```python
from build123d import *

# Parameters (mm, degrees)
SKETCH1_R           = 48.26
SKETCH1_R_2         = 1.1303
SKETCH1_R_3         = 17.4625
SKETCH1_R_4         = 3.175
BOSS_EXTRUDE1_DEPTH = 3.175


with BuildPart() as part:
    # Sketch1 → Boss-Extrude1 (new body)
    with BuildSketch(Plane(origin=(0, 0, 0), x_dir=(0, 0, -1), z_dir=(1, 0, 0))):
        Circle(SKETCH1_R)
        with Locations((0, 45.085)):
            Circle(SKETCH1_R_2, mode=Mode.SUBTRACT)
        with Locations((31.87990923, 31.87990923)):
            Circle(SKETCH1_R_2, mode=Mode.SUBTRACT)
        with Locations((45.085, 0)):
            Circle(SKETCH1_R_2, mode=Mode.SUBTRACT)
        with Locations((31.87990923, -31.87990923)):
            Circle(SKETCH1_R_2, mode=Mode.SUBTRACT)
        with Locations((0, -45.085)):
            Circle(SKETCH1_R_2, mode=Mode.SUBTRACT)
        with Locations((-31.87990923, -31.87990923)):
            Circle(SKETCH1_R_2, mode=Mode.SUBTRACT)
        with Locations((-45.085, 0)):
            Circle(SKETCH1_R_2, mode=Mode.SUBTRACT)
        with Locations((-31.87990923, 31.87990923)):
            Circle(SKETCH1_R_2, mode=Mode.SUBTRACT)
        Circle(SKETCH1_R_3, mode=Mode.SUBTRACT)
        with Locations((9.720159182, 23.466540126)):
            Circle(SKETCH1_R_4, mode=Mode.SUBTRACT)
        with Locations((23.466540126, -9.720159182)):
            Circle(SKETCH1_R_4, mode=Mode.SUBTRACT)
        with Locations((-9.720159182, -23.466540126)):
            Circle(SKETCH1_R_4, mode=Mode.SUBTRACT)
        with Locations((-23.466540126, 9.720159182)):
            Circle(SKETCH1_R_4, mode=Mode.SUBTRACT)
    extrude(amount=BOSS_EXTRUDE1_DEPTH)


solid = part.part
```
Check sheet for the modelled part. Datum: model origin and axes. Units: mm. Round coordinates to 2 decimals unless told otherwise and drop trailing zeros. Loops run counter-clockwise (first coordinate to the right, second up) from the corner with the lowest first, then second, coordinate; pieces in that order, holes last. Notation, with made-up numbers: (-17, -1.5) -> (2, -1.5) arc R18 cw to (2, 28.5) -> close; hole circle Ø8 at (38, 27.25). An arc over 180 degrees is marked (long way). Write item = value, one per line. Start each with the question number.
1) Sectioned sample at D-D, the plane z = -23.5. Record the cut outline in (x, y) (3 decimals).
2) Release check for a two-part mould opening along Y. For faces 1 (the flat face through (0, -21, 1)), 2 (the cylindrical face through (1.57, 14.5, -46.03)), 3 (the cylindrical face through (1.57, -30.93, 31.27)), 4 (the cylindrical face through (1.565, -43.964, 0.147)) record: released by +Y, released by -Y, zero draft, split by the parting line, or undercut.
3) Gauge pin test, flat ends, axial feed: pin 1 Ø2 at (y, z) = (-31.88, -31.88) entering from +X; pin 2 Ø1.5 at (x, y) = (2.5, 21.5) entering from -Z; pin 3 Ø1 at (x, y) = (2, 15.5) entering from -Z. Record the tip position at first contact, or that the pin passes through.
4) Sectioned sample at A-A, the plane z = 0. Record the cut outline in (x, y) (1 decimal).
5) Sectioned sample at C-C, the plane x = 2.2. State how many separate pieces and enclosed holes the cut face has, plus the area to 3 significant figures.
6) Thickness scan on probe 1 along Y at (x, z) = (1.9, 0); probe 2 along Y at (x, z) = (2.3, 31); probe 3 along Z at (x, y) = (2.15, -7.5). Record the ranges inside material, lowest first.
Results are:
q1.outline = (0, -42.152) -> (3.175, -42.152) -> (3.175, -12.895) -> (0, -12.895) -> close; (0, -6.545) -> (3.175, -6.545) -> (3.175, 42.152) -> (0, 42.152) -> close
q2.face_1 = zero draft
q2.face_2 = split by the parting line
q2.face_3 = undercut
q2.face_4 = undercut
q3.pin_1 = through
q3.pin_2 = -43.57
q3.pin_3 = -45.87
q4.outline = (0, -48.3) -> (3.2, -48.3) -> (3.2, -46.2) -> (0, -46.2) -> close; (0, -44) -> (3.2, -44) -> (3.2, -17.5) -> (0, -17.5) -> close; (0, 17.5) -> (3.2, 17.5) -> (3.2, 44) -> (0, 44) -> close; (0, 46.2) -> (3.2, 46.2) -> (3.2, 48.3) -> (0, 48.3) -> close
q5.separate_pieces = 1
q5.enclosed_holes = 13
q5.area = 6,200 mm^2
q6.probe_1 = -48.26 to -46.22, -43.95 to -17.46, 17.46 to 43.95, 46.22 to 48.26
q6.probe_2 = -36.99 to -32.59, -31.17 to 31.17, 32.59 to 36.99
q6.probe_3 = -47.67 to -25.74, -21.2 to -15.77, 15.77 to 47.67
